Part model, mm, in its own coordinate system. A direction names the side the tool comes from. Give positions to 0.01 mm unless a question says otherwise; leave off trailing zeros. Loops run counter-clockwise (first coordinate to the right, second up) from the corner with the lowest first, then second, coordinate; pieces in that order, holes last. Notation, with made-up numbers: M 63,0 L 72,0 A31 ccw 72,31 Z; hole C 33,-1 d9. An arc over 180 degrees is marked long. Put each result on its own line as item: value. Start each with the question number.
```python
from build123d import *

# Parameters (mm, degrees)
BOSS_EXTRUDE1_DEPTH                                 = 6.35
CBORE_FOR_00_BINDING_HEAD_MACHINE_SCREW_D           = 3.000000096
CBORE_FOR_00_BINDING_HEAD_MACHINE_SCREW_CBORE_D     = 5.999999938
CBORE_FOR_00_BINDING_HEAD_MACHINE_SCREW_CBORE_DEPTH = 3.000000096
SKETCH6_W                                           = 12.7
SKETCH6_H                                           = 15.875
CUT_EXTRUDE1_DEPTH                                  = 6.35
FILLET2_R                                           = 2.54
CBORE_FOR_00_BINDING_HEAD_MACHINE_S_2_D             = 11.999999876
CBORE_FOR_00_BINDING_HEAD_MACHINE_S_2_CBORE_D       = 16.000000004
CBORE_FOR_00_BINDING_HEAD_MACHINE_S_2_CBORE_DEPTH   = 3.999999874


with BuildPart() as part:
    # Sketch1 → Boss-Extrude1 (new body)
    with BuildSketch(Plane.XY):
        with BuildLine():
            Line((-57.15, 31.75), (57.15, 31.75))
            ThreePointArc((57.15, 31.75), (70.620384182, 26.170384182), (76.2, 12.7))
            Line((76.2, 12.7), (76.2, -12.7))
            ThreePointArc((76.2, -12.7), (70.620384182, -26.170384182), (57.15, -31.75))
            Line((57.15, -31.75), (-57.15, -31.75))
            ThreePointArc((-57.15, -31.75), (-70.620384182, -26.170384182), (-76.2, -12.7))
            Line((-76.2, -12.7), (-76.2, 12.7))
            ThreePointArc((-76.2, 12.7), (-70.620384182, 26.170384182), (-57.15, 31.75))
        make_face()
    extrude(amount=BOSS_EXTRUDE1_DEPTH)

    # CBORE for _00 Binding Head Machine Screw (through all)
    with Locations(Plane.XY.offset(6.35)):
        with Locations((-20, 25.65), (20, 25.65), (3.81, -27.94), (-3.81, -27.94)):
            CounterBoreHole(CBORE_FOR_00_BINDING_HEAD_MACHINE_SCREW_D / 2, CBORE_FOR_00_BINDING_HEAD_MACHINE_SCREW_CBORE_D / 2, CBORE_FOR_00_BINDING_HEAD_MACHINE_SCREW_CBORE_DEPTH)

    # Sketch6 → Cut-Extrude1 (cut)
    with BuildSketch(Plane(origin=(0, 0, 0), x_dir=(-1, 0, 0), z_dir=(0, 0, -1))):
        with Locations((-25.4, -23.8125)):
            Rectangle(SKETCH6_W, SKETCH6_H)
        with Locations((25.4, -23.8125)):
            Rectangle(SKETCH6_W, SKETCH6_H)
    extrude(amount=-CUT_EXTRUDE1_DEPTH, mode=Mode.SUBTRACT)

    # Fillet2
    fillet2_edges = [part.edges().sort_by_distance(p)[0] for p in [
        (19.05, -15.875, 3.175),
        (31.75, -15.875, 3.175),
        (-19.05, -15.875, 3.175),
        (-31.75, -15.875, 3.175),
    ]]
    fillet(fillet2_edges, radius=FILLET2_R)

    # CBORE for _00 Binding Head Machine S 2 (through all)
    with Locations(Plane(origin=(0, 0, 0), x_dir=(1, 0, 0), z_dir=(0, 0, -1))):
        with Locations((-60.325, -6.35), (60.325, -6.35)):
            CounterBoreHole(CBORE_FOR_00_BINDING_HEAD_MACHINE_S_2_D / 2, CBORE_FOR_00_BINDING_HEAD_MACHINE_S_2_CBORE_D / 2, CBORE_FOR_00_BINDING_HEAD_MACHINE_S_2_CBORE_DEPTH)


solid = part.part
```
1) Band-saw the part on B-B on x = -3.81. Give the cut face in (y, z), then the cut area to 3 significant figures.
2) Band-saw the part on D-D on x = -25.5. Give the cut face in (y, z) (3 decimals), then the cut area to 3 significant figures.
3) Band-saw the part on C-C on y = 25.65. Give the cut face in (x, z).
4) Wall check: L1, parallel to Y at x = -3.81, z = 4.6; L2, parallel to X at y = -19, z = 5; L3, parallel to Y at x = 3.81, z = 2.2. Give the ranges that are in metal, low to high.
5) Band-saw the part on A-A on z = 1.5. Give the cut face in (x, y) (3 decimals).
6) Which spindle directions (+Z, -Z, +X, -X, +Y, -Y) get a long thin tool onto all of the face, cutting with end or side? Do faces 1 (the flat face through (-76.2, 0, 3)), 2 (the flat face through (21, 27, 3.35)), 3 (the cylindrical face through (30.986, -16.599, 3.219)), 4 (the cylindrical face through (-52.935, 9.414, 1.972)), 5 (the cylindrical face through (-70.47, -26.32, 3.13)). Say none if no direction does.
7) Pin check, flat tips, straight feed: pin 1 Ø1.5 at (y, z) = (-23, 5) entering from -X; pin 2 Ø1.9 at (x, z) = (26, 2.5) entering from -Y (3 decimals); pin 3 Ø1 at (y, z) = (-14.5, 4) entering from -X. Stop position of each tip, or through.
Evaluation:
1. outline: M -31.75,0 L -29.44,0 L -29.44,3.35 L -30.94,3.35 L -30.94,6.35 L -31.75,6.35 Z; M -26.44,0 L 31.75,0 L 31.75,6.35 L -24.94,6.35 L -24.94,3.35 L -26.44,3.35 Z
1. area: 375 mm2
2. outline: M -15.875,0 L 31.75,0 L 31.75,6.35 L -15.875,6.35 Z
2. area: 302 mm2
3. outline: M -71.12,0 L -21.5,0 L -21.5,3.35 L -23,3.35 L -23,6.35 L -71.12,6.35 Z; M -18.5,0 L 18.5,0 L 18.5,3.35 L 17,3.35 L 17,6.35 L -17,6.35 L -17,3.35 L -18.5,3.35 Z; M 21.5,0 L 71.12,0 L 71.12,6.35 L 23,6.35 L 23,3.35 L 21.5,3.35 Z
4. L1: -31.75 to -30.94, -24.94 to 31.75
4. L2: -75.13 to -31.75, -19.05 to 19.05, 31.75 to 75.13
4. L3: -31.75 to -29.44, -26.44 to 31.75
5. outline: M -76.2,-12.7 A19.05 ccw -57.15,-31.75 L -31.75,-31.75 L -31.75,-18.415 A2.54 cw -29.21,-15.875 L -21.59,-15.875 A2.54 cw -19.05,-18.415 L -19.05,-31.75 L 19.05,-31.75 L 19.05,-18.415 A2.54 cw 21.59,-15.875 L 29.21,-15.875 A2.54 cw 31.75,-18.415 L 31.75,-31.75 L 57.15,-31.75 A19.05 ccw 76.2,-12.7 L 76.2,12.7 A19.05 ccw 57.15,31.75 L -57.15,31.75 A19.05 ccw -76.2,12.7 Z; hole C -60.325,6.35 d16; hole C -20,25.65 d3; hole C -3.81,-27.94 d3; hole C 3.81,-27.94 d3; hole C 20,25.65 d3; hole C 60.325,6.35 d16
6. face 1: +Z, -Z, -X, +Y, -Y
6. face 2: +Z
6. face 3: +Z, -Z, -Y
6. face 4: -Z
6. face 5: +Z, -Z, -X, -Y
7. pin 1: x = -73.63
7. pin 2: y = -15.875
7. pin 3: x = -76.16
